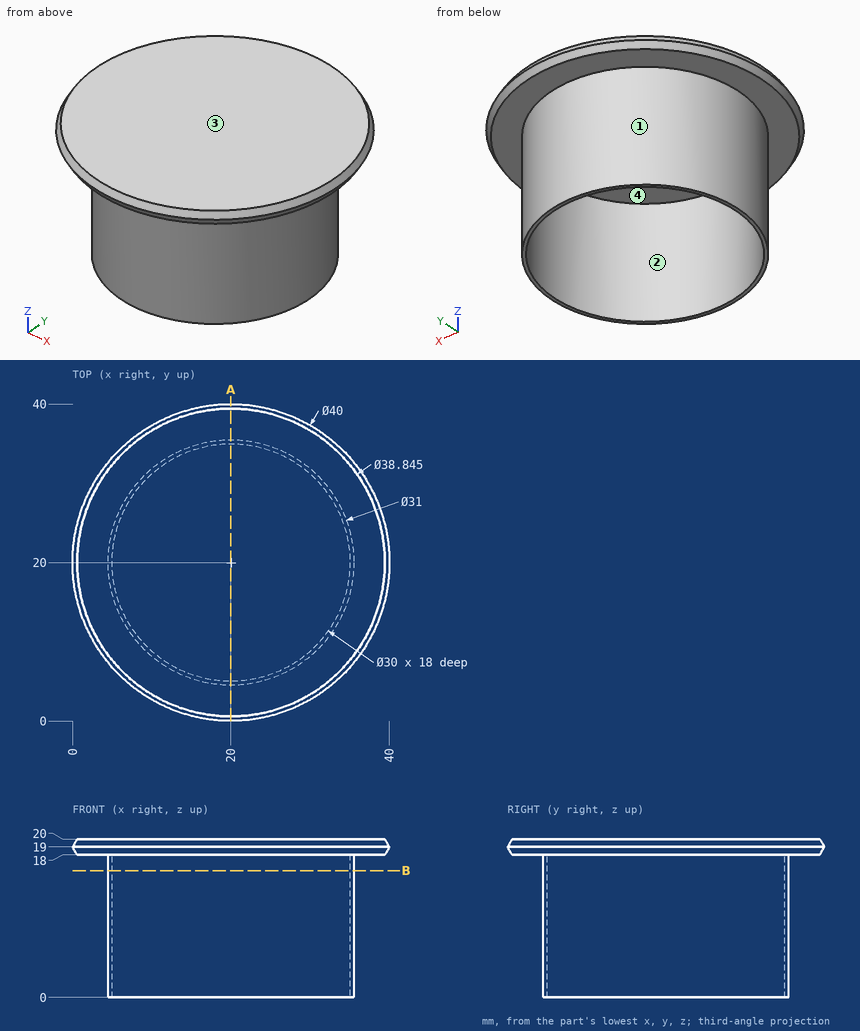
Print and shaded views of the part. All mm, measured from the part's lowest x, y and z. Give positions to 0.01 mm unless a question says otherwise; leave off trailing zeros. Loops run counter-clockwise (first coordinate to the right, second up) from the corner with the lowest first, then second, coordinate; pieces in that order, holes last. Notation, with made-up numbers: (-10.5, 52.5) -> (31.5, 52.5) arc R14 ccw to (31.5, 65.5) -> close; hole circle Ø2 at (-40, 76). An arc over 180 degrees is marked (long way). Use CSV: the item, a comma, the result in double quotes. Start each with the question number.
1) Slice it at A-A on x = 20. Give the cut face in (y, z).
2) Slice it at B-B on z = 16. Give the cut face in (x, y).
3) Flat gauge pins, fed straight in: pin 1 Ø2 at (x, z) = (23.5, 10) entering from +Y; pin 2 Ø4 at (x, y) = (29.5, 10.5) entering from -Z; pin 3 Ø3 at (y, z) = (13.5, 8) entering from -X; pin 4 Ø1 at (x, z) = (11, 9) entering from +Y. Where does each tip first touch, or does it go through?
4) Wall check: line 1 (Y direction, x = 20, z = 5.25); line 2 (Z direction, x = 29, y = 13); line 3 (Y direction, x = 26.5, z = 5.75). Give the ranges that are in metal, low to high.
5) Mould opens along X. For the marked faces 1, 2, 3 and 4 say: released by +X, released by -X, zero draft, split by the parting line, or undercut.
Computed values:
1,outline,"(0, 19) -> (0.58, 18) -> (4.5, 18) -> (4.5, 0) -> (5, 0) -> (5, 18) -> (35, 18) -> (35, 0) -> (35.5, 0) -> (35.5, 18) -> (39.42, 18) -> (40, 19) -> (39.42, 20) -> (0.58, 20) -> close"
2,outline,"circle Ø31 at (20, 20); hole circle Ø30 at (20, 20)"
3,pin 1,"stops at y = 35.3"
3,pin 2,"stops at z = 0"
3,pin 3,"stops at x = 5.33"
3,pin 4,"stops at y = 32.96"
4,line 1,"y = 4.5 to 5, 35 to 35.5"
4,line 2,"z = 18 to 20"
4,line 3,"y = 5.93 to 6.48, 33.52 to 34.07"
5,face 1,"split by the parting line"
5,face 2,"undercut"
5,face 3,"zero draft"
5,face 4,"undercut"
